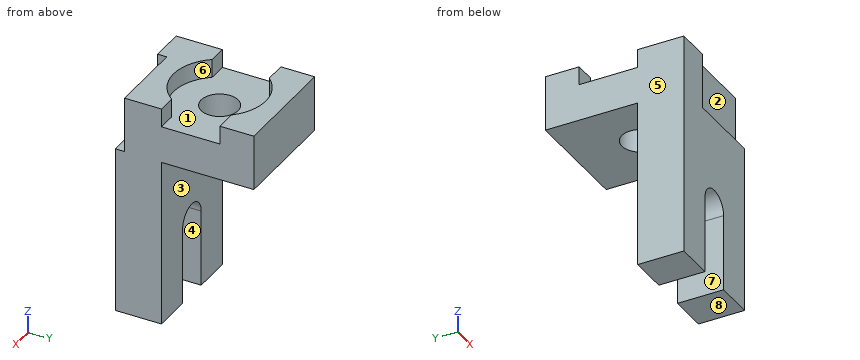
```python
from build123d import *

# Parameters (mm, degrees)
SKETCH1_R           = 12
BOSS_EXTRUDE1_DEPTH = 24
BOSS_EXTRUDE2_DEPTH = 36
SKETCH1_9_W         = 72
SKETCH1_9_H         = 30
BOSS_EXTRUDE5_DEPTH = 109
SKETCH1_10_W        = 50
SKETCH1_10_H        = 6
BOSS_EXTRUDE6_DEPTH = 36
CUT_EXTRUDE1_DEPTH  = 30


with BuildPart() as part:
    # Sketch1 → Boss-Extrude1 (new body)
    # profile 1 of 5: a face of its own
    with BuildSketch(Plane.XY):
        with BuildLine():
            Line((22.360679775, 23), (-22.360679775, 23))
            ThreePointArc((-22.360679775, 23), (-29.972123003, 4.292997564), (-24, -15))
            Line((-24, -15), (24, -15))
            ThreePointArc((24, -15), (28.460498942, -6.486832981), (30, 3))
            ThreePointArc((30, 3), (28.025170769, 13.704662693), (22.360679775, 23))
        make_face()
        with Locations((0, 3)):
            Circle(SKETCH1_R, mode=Mode.SUBTRACT)
    # profile 2 of 5: a face of its own
    with BuildSketch(Plane.XY):
        with BuildLine():
            ThreePointArc((22.360679775, 23), (0, 33), (-22.360679775, 23))
            Line((-22.360679775, 23), (22.360679775, 23))
        make_face()
    # profile 3 of 5: a face of its own
    with BuildSketch(Plane.XY):
        with BuildLine():
            Line((24, -15), (-24, -15))
            ThreePointArc((-24, -15), (0, -27), (24, -15))
        make_face()
    # profile 4 of 5: a face of its own
    with BuildSketch(Plane.XY):
        with BuildLine():
            Line((36, -15), (36, 23))
            Line((36, 23), (22.360679775, 23))
            ThreePointArc((22.360679775, 23), (28.025170769, 13.704662693), (30, 3))
            ThreePointArc((30, 3), (28.460498942, -6.486832981), (24, -15))
            Line((24, -15), (36, -15))
        make_face()
    # profile 5 of 5: a face of its own
    with BuildSketch(Plane.XY):
        with BuildLine():
            Line((-22.360679775, 23), (-36, 23))
            Line((-36, 23), (-36, -15))
            Line((-36, -15), (-24, -15))
            ThreePointArc((-24, -15), (-29.972123003, 4.292997564), (-22.360679775, 23))
        make_face()
    extrude(amount=BOSS_EXTRUDE1_DEPTH)

    # Sketch1<4> → Boss-Extrude2 (add)
    with BuildSketch(Plane.XY):
        with BuildLine():
            Line((36, 45), (-36, 45))
            Line((-36, 45), (-36, 23))
            Line((-36, 23), (-22.360679775, 23))
            ThreePointArc((-22.360679775, 23), (0, 33), (22.360679775, 23))
            Line((22.360679775, 23), (36, 23))
            Line((36, 23), (36, 45))
        make_face()
        with BuildLine():
            Line((-24, -15), (-36, -15))
            Line((-36, -15), (-36, -45))
            Line((-36, -45), (-14, -45))
            Line((-14, -45), (-14, -39))
            Line((-14, -39), (36, -39))
            Line((36, -39), (36, -15))
            Line((36, -15), (24, -15))
            ThreePointArc((24, -15), (0, -27), (-24, -15))
        make_face()
    extrude(amount=BOSS_EXTRUDE2_DEPTH)

    # Sketch1<9> → Boss-Extrude5 (add)
    with BuildSketch(Plane.XY):
        with Locations((0, -30)):
            Rectangle(SKETCH1_9_W, SKETCH1_9_H)
    extrude(amount=-BOSS_EXTRUDE5_DEPTH)

    # Sketch1<10> → Boss-Extrude6 (add)
    with BuildSketch(Plane.XY):
        with Locations((11, -42)):
            Rectangle(SKETCH1_10_W, SKETCH1_10_H)
    extrude(amount=-BOSS_EXTRUDE6_DEPTH)

    # Sketch3 → Cut-Extrude1 (cut)
    with BuildSketch(Plane(origin=(0, -15, 0), x_dir=(1, 0, 0), z_dir=(0, 1, 0))):
        with BuildLine():
            Line((11, 59), (11, 109))
            Line((11, 109), (-11, 109))
            Line((-11, 109), (-11, 59))
            ThreePointArc((-11, 59), (0, 70), (11, 59))
        make_face()
        with BuildLine():
            ThreePointArc((-11, 59), (0, 48), (11, 59))
            Line((11, 59), (-11, 59))
        make_face()
        with BuildLine():
            Line((-11, 59), (11, 59))
            ThreePointArc((11, 59), (0, 70), (-11, 59))
        make_face()
    extrude(amount=-CUT_EXTRUDE1_DEPTH, mode=Mode.SUBTRACT)


solid = part.part
```
The model under review builds one solid part; all positions refer to its coordinate system, in mm. Face numbers are marked on the shaded views. A direction names the side the tool comes from. Give positions to 0.01 mm unless a question says otherwise; leave off trailing zeros. Loops run counter-clockwise (first coordinate to the right, second up) from the corner with the lowest first, then second, coordinate; pieces in that order, holes last. Notation, with made-up numbers: (33, 37.25) - (49, 37.25) arc R15 cw to (49, 56.25) - close; hole circle Ø8 at (66, 22.25). An arc over 180 degrees is marked (long way). Answer as a JSON object with one key per item and string values.
Q1. For the marked faces 1, 2, 3 and 4, list the 3-axis set-ups (+Z, -Z, +X, -X, +Y, -Y) from which the entire face can be reached by the end or side of a thin tool; tool diameter is ignored.
Worked out:
{"face 1": "+Z", "face 2": "+Z, +X, -Y", "face 3": "-Z, +X, -X, +Y", "face 4": "-Z, +Y, -Y"}
Q2. Add section B-B on z = 25.5. State the section outline as (x, y) points, plus the area to 3 significant figures.
Worked out:
{"outline": "(-36, -45) - (-14, -45) - (-14, -39) - (36, -39) - (36, -15) - (24, -15) arc R30 cw to (-24, -15) - (-36, -15) - close; (-36, 23) - (-22.36, 23) arc R30 cw to (22.36, 23) - (36, 23) - (36, 45) - (-36, 45) - close", "area": "2,730 mm^2"}
Q3. To check wall thickness, follow line 1 along Y through (x, z) = (0, 6.75); line 2 along Z through (x, y) = (-17.5, 24); line 3 along Z through (x, y) = (15.5, 29). State the ranges of each line that lie inside material, in increasing order.
Worked out:
{"line 1": "y = -39 to -9, 15 to 45", "line 2": "z = 0 to 24", "line 3": "z = 0 to 36"}
Q4. Add section C-C on x = 0. State the section outline as (y, z) points.
Worked out:
{"outline": "(-45, -48) - (-15, -48) - (-15, 0) - (-9, 0) - (-9, 24) - (-27, 24) - (-27, 36) - (-39, 36) - (-39, 0) - (-45, 0) - close; (15, 0) - (45, 0) - (45, 36) - (33, 36) - (33, 24) - (15, 24) - close"}
Q5. Add section A-A on y = 3. State the section outline as (x, z) points.
Worked out:
{"outline": "(-36, 0) - (-12, 0) - (-12, 24) - (-36, 24) - close; (12, 0) - (36, 0) - (36, 24) - (12, 24) - close"}
Q6. Add section D-D on z = 4.5. State the section outline as (x, y) points, plus the area to 3 significant figures.
Worked out:
{"outline": "(-36, -45) - (-14, -45) - (-14, -39) - (36, -39) - (36, 45) - (-36, 45) - close; hole circle Ø24 at (0, 3)", "area": "5,730 mm^2"}
Q7. Mouldability with a two-part tool opening along X and no side actions: class the marked faces 5, 6, 7 and 8 as +X half, -X half, draft (parallel to the pull), parting line (faces both ways), or undercut.
Worked out:
{"face 5": "-X half", "face 6": "undercut", "face 7": "undercut", "face 8": "draft"}
Q8. Insertion check: pin 1 (18 mm diameter, centred on x = -13.5, y = -3, fed in from +Z); pin 2 (5 mm diameter, centred on y = -41, z = 12, fed in from +X); pin 3 (6 mm diameter, centred on x = 23.5, y = 29.5, fed in from -Z); pin 4 (8 mm diameter, centred on x = 14, z = -40.5, fed in from +Y). Each pin has a flat end and moves straight along its axis. Give the tip position at first contact, or say it passes through.
Worked out:
{"pin 1": "stops at z = 24", "pin 2": "stops at x = 36", "pin 3": "stops at z = 0", "pin 4": "stops at y = -15"}
